The listing builds one solid part. Answer for the finished solid, in the listing's coordinates (mm). Face numbers are marked on the shaded views. A direction names the side the tool comes from. Coordinates: 2 decimals unless noted, no trailing zeros. Order: outer loops, then holes, each group sorted by start corner. A loop starts at its lowest first (then second) coordinate and runs counter-clockwise, first axis right, second up. Notation, with made-up numbers: (19.25, 31.25) -> (49.25, 31.25) arc R10 cw to (49.25, 40.25) -> close; hole circle Ø2 at (1, 1.5). An arc over 180 degrees is marked (long way). Return JSON: item names as keys, results as strings.
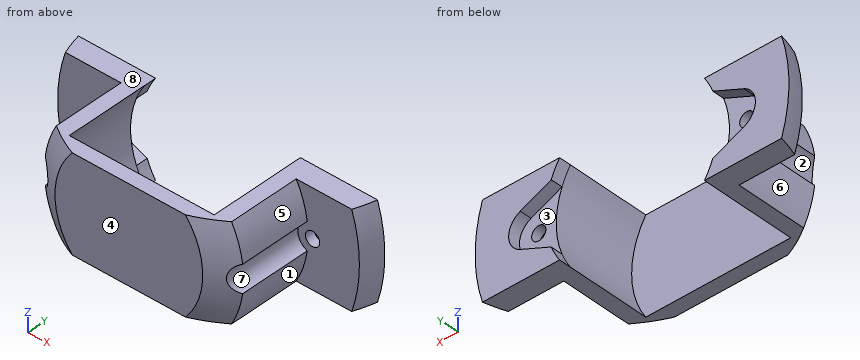
```python
from build123d import *

# Parameters (mm, degrees)
SKETCH2_R               = 33.8
CUT_EXTRUDE1_DEPTH      = 7
SKETCH3_OUTSIDE_W       = 87.592
SKETCH3_OUTSIDE_H       = 87.592
SKETCH3_OUTSIDE_W_2     = 66.134408594
SKETCH3_OUTSIDE_H_2     = 20
CUT_EXTRUDE2_DEPTH      = 54.899165114
CUT_EXTRUDE3_DEPTH      = 2.5
SKETCH6_R               = 18.25
SKETCH6_R_2             = 1.5
CUT_EXTRUDE4_DEPTH      = 17.5
CUT_EXTRUDE5_START      = -19.484712572
CUT_EXTRUDE5_DEPTH      = 14.984712572
CUT_EXTRUDE6_START      = -3
SKETCH8_R               = 33.067204297
CUT_EXTRUDE6_DEPTH      = 37.917915802
CUT_EXTRUDE7_REACH      = 41.188
CUT_EXTRUDE7_END_RADIUS = 33.8
SKETCH9_R               = 3.1


# Read off the part's stored shape, not the designer's step: Cut-Extrude5
with BuildPart() as part:
    # Sketch1 → Revolve1 (revolve)
    with BuildSketch(Plane.XY, mode=Mode.PRIVATE) as revolve1_sk:
        with BuildLine():
            Line((0, -33.8), (0, 0))
            Line((0, 0), (33.8, 0))
            ThreePointArc((33.8, 0), (23.900209204, -23.900209204), (0, -33.8))
        make_face()
    revolve(revolve1_sk.sketch.rotate(Axis((0, -33.8, 0), (0, 1, 0)), 180), axis=Axis((0, -33.8, 0), (0, 1, 0)))

    # Sketch2 → Cut-Extrude1 (cut)
    with BuildSketch(Plane(origin=(0, 0, 0), x_dir=(1, 0, 0), z_dir=(0, 1, 0))):
        Circle(SKETCH2_R)
    extrude(amount=-CUT_EXTRUDE1_DEPTH, mode=Mode.SUBTRACT)

    # Sketch3 outside → Cut-Extrude2 (cut, through all)
    with BuildSketch(Plane(origin=(0, -7, 0), x_dir=(1, 0, 0), z_dir=(0, 1, 0))):
        Rectangle(SKETCH3_OUTSIDE_W, SKETCH3_OUTSIDE_H)
        Rectangle(SKETCH3_OUTSIDE_W_2, SKETCH3_OUTSIDE_H_2, mode=Mode.SUBTRACT)
    extrude(amount=-CUT_EXTRUDE2_DEPTH, mode=Mode.SUBTRACT)

    # Sketch5 → Cut-Extrude3 (cut)
    with BuildSketch(Plane(origin=(0, -7, 0), x_dir=(1, 0, 0), z_dir=(0, 1, 0))):
        with BuildLine():
            Line((-17.025732229, 6.571677263), (-23.544283672, 3.742739979))
            ThreePointArc((-23.544283672, 3.742739979), (-26, 0), (-23.544283672, -3.742739979))
            Line((-23.544283672, -3.742739979), (-17.025732229, -6.571677263))
            ThreePointArc((-17.025732229, -6.571677263), (0, -18.25), (17.025732229, -6.571677263))
            Line((17.025732229, -6.571677263), (23.544283672, -3.742739979))
            ThreePointArc((23.544283672, -3.742739979), (26, 0), (23.544283672, 3.742739979))
            Line((23.544283672, 3.742739979), (17.025732229, 6.571677263))
            ThreePointArc((17.025732229, 6.571677263), (0, 18.25), (-17.025732229, 6.571677263))
        make_face()
    extrude(amount=-CUT_EXTRUDE3_DEPTH, mode=Mode.SUBTRACT)

    # Sketch6 → Cut-Extrude4 (cut)
    with BuildSketch(Plane(origin=(0, -9.5, 0), x_dir=(1, 0, 0), z_dir=(0, 1, 0))):
        Circle(SKETCH6_R)
        with Locations(Location((-21.92, 0, 0), (0, 0, 270))):
            Circle(SKETCH6_R_2)
        with Locations(Location((21.92, 0, 0), (0, 0, 270))):
            Circle(SKETCH6_R_2)
    extrude(amount=-CUT_EXTRUDE4_DEPTH, mode=Mode.SUBTRACT)

    # Cut-Extrude5 outline → Cut-Extrude5 (cut)
    with BuildSketch(Plane(origin=(0, -7, 0), x_dir=(1, 0, 0), z_dir=(0, 1, 0)).offset(CUT_EXTRUDE5_START)):
        with BuildLine():
            ThreePointArc((20.967983577, -1.159165532), (20.206521411, -5.718084686), (18.466185313, -10))
            Line((18.466185313, -10), (33, -10))
            Line((33, -10), (33, 10))
            Line((33, 10), (18.466185313, 10))
            ThreePointArc((18.466185313, 10), (20.206521411, 5.718084686), (20.967983577, 1.159165532))
            ThreePointArc((20.967983577, 1.159165532), (23.42, 0), (20.967983577, -1.159165532))
        make_face()
        with BuildLine():
            ThreePointArc((-18.466185313, -10), (-20.206521411, -5.718084686), (-20.967983577, -1.159165532))
            ThreePointArc((-20.967983577, -1.159165532), (-23.42, 0), (-20.967983577, 1.159165532))
            ThreePointArc((-20.967983577, 1.159165532), (-20.206521411, 5.718084686), (-18.466185313, 10))
            Line((-18.466185313, 10), (-33, 10))
            Line((-33, 10), (-33, -10))
            Line((-33, -10), (-18.466185313, -10))
        make_face()
    extrude(amount=CUT_EXTRUDE5_DEPTH, mode=Mode.SUBTRACT)

    # Sketch8 → Cut-Extrude6 (cut, through all)
    with BuildSketch(Plane(origin=(0, -27, 0), x_dir=(1, 0, 0), z_dir=(0, 1, 0)).offset(CUT_EXTRUDE6_START)):
        Circle(SKETCH8_R)
    extrude(amount=-CUT_EXTRUDE6_DEPTH, mode=Mode.SUBTRACT)

    # Cut-Extrude7: up to this sphere (the profile starts inside it)
    cut_extrude7_end = Location((0, 0, 0)) * Sphere(CUT_EXTRUDE7_END_RADIUS, mode=Mode.PRIVATE)
    # Sketch9 → Cut-Extrude7 (cut, up to the surface)
    with BuildSketch(Plane.XZ.offset(11.5), mode=Mode.PRIVATE) as cut_extrude7_sk1:
        with Locations((-21.92, 0)):
            Circle(SKETCH9_R)
    cut_extrude7_tool1 = extrude(cut_extrude7_sk1.sketch, amount=CUT_EXTRUDE7_REACH, mode=Mode.PRIVATE) & cut_extrude7_end
    add(cut_extrude7_tool1.solids().sort_by_distance((-21.92, -11.5, 0))[0], mode=Mode.SUBTRACT)
    # Sketch9 → Cut-Extrude7 (cut, up to the surface)
    with BuildSketch(Plane.XZ.offset(11.5), mode=Mode.PRIVATE) as cut_extrude7_sk2:
        with Locations((21.92, 0)):
            Circle(SKETCH9_R)
    cut_extrude7_tool2 = extrude(cut_extrude7_sk2.sketch, amount=CUT_EXTRUDE7_REACH, mode=Mode.PRIVATE) & cut_extrude7_end
    add(cut_extrude7_tool2.solids().sort_by_distance((21.92, -11.5, 0))[0], mode=Mode.SUBTRACT)


solid = part.part
```
Item 1: Determine the mould class of the marked faces 6, 7 and 8 for opening direction Z: pulls with the +Z half, pulls with the -Z half, needs draft (parallel to the pull), parting line crosses it, or undercut.
Answer list:
{"face 6": "pulls with the -Z half", "face 7": "undercut", "face 8": "pulls with the +Z half"}
Item 2: The part is cut by section C-C on x = 21.92. Determine the outline of the cut face in (y, z).
Answer list:
{"outline": "(-11.5, -10) -> (-7, -10) -> (-7, -4.45) -> (-9.5, -4.45) -> (-9.5, -1.5) -> (-11.5, -1.5) -> close; (-11.5, 1.5) -> (-9.5, 1.5) -> (-9.5, 4.45) -> (-7, 4.45) -> (-7, 10) -> (-11.5, 10) -> close"}
Item 3: The part is cut by section D-D on z = -4.75. Determine the outline of the cut face in (x, y), plus the area to 3 significant figures.
Answer list:
{"outline": "(-32.72, -7) arc R33.46 ccw to (-31.43, -11.5) -> (-20.46, -11.5) -> (-20.46, -26.48) arc R33.46 ccw to (-14.83, -30) -> (14.83, -30) arc R33.46 ccw to (20.46, -26.48) -> (20.46, -11.5) -> (31.43, -11.5) arc R33.46 ccw to (32.72, -7) -> (21.22, -7) -> (21.22, -9.5) -> (17.62, -9.5) -> (17.62, -27) -> (-17.62, -27) -> (-17.62, -9.5) -> (-21.22, -9.5) -> (-21.22, -7) -> close", "area": "305 mm2"}
Item 4: The part is cut by section B-B on z = 0. Determine the outline of the cut face in (x, y), plus the area to 3 significant figures.
Answer list:
{"outline": "(-33.07, -7) arc R33.8 ccw to (-31.78, -11.5) -> (-23.42, -11.5) -> (-23.42, -9.5) -> (-26, -9.5) -> (-26, -7) -> close; (-20.42, -11.5) -> (-18.82, -11.5) -> (-18.82, -28.08) arc R33.8 ccw to (-15.57, -30) -> (15.57, -30) arc R33.8 ccw to (18.82, -28.08) -> (18.82, -11.5) -> (20.42, -11.5) -> (20.42, -9.5) -> (18.25, -9.5) -> (18.25, -27) -> (-18.25, -27) -> (-18.25, -9.5) -> (-20.42, -9.5) -> close; (23.42, -11.5) -> (31.78, -11.5) arc R33.8 ccw to (33.07, -7) -> (26, -7) -> (26, -9.5) -> (23.42, -9.5) -> close", "area": "202 mm2"}
Item 5: Flat-ended cylindrical pins translate along their axes: pin 1 (10 mm diameter, centred on x = 25, z = 7, fed in from -Y); pin 2 (2.5 mm diameter, centred on x = 21, z = -0.5, fed in from +Y); pin 3 (5 mm diameter, centred on y = -15.5, z = 7, fed in from -X); pin 4 (2 mm diameter, centred on x = 2, y = -24.5, fed in from +Z). Find the tip coordinate at first contact, or state that the pin passes through.
Answer list:
{"pin 1": "y = -26.52", "pin 2": "y = -9.5", "pin 3": "x = -20.51", "pin 4": "through"}
Item 6: The part is cut by section A-A on y = -19.75. Determine the outline of the cut face in (x, z).
Answer list:
{"outline": "(-20.8, -2.89) arc R21 ccw to (-18.47, -10) -> (-15.27, -10) arc R18.25 cw to (-15.27, 10) -> (-18.47, 10) arc R21 ccw to (-20.8, 2.89) arc R3.1 cw to start; (15.27, -10) -> (18.47, -10) arc R21 ccw to (20.8, -2.89) arc R3.1 cw to (20.8, 2.89) arc R21 ccw to (18.47, 10) -> (15.27, 10) arc R18.25 cw to start"}
Item 7: Which of the six approach directions +Z, -Z, +X, -X, +Y, -Y give full straight-line access (tool end or side, diameter ignored) to the marked faces 1, 2, 3, 4 and 5?
Answer list:
{"face 1": "-Z, +X, -Y", "face 2": "-X, -Y", "face 3": "+Y", "face 4": "+Z, -Z, +X, -X, -Y", "face 5": "+Z, +X, -Y"}
Item 8: Find the intervals of material crossed by probe 1 along Z at (x, y) = (-21.92, -10.7); probe 2 along X at (y, z) = (-11, 0); probe 3 along Y at (x, z) = (11, -7), in increasing order.
Answer list:
{"probe 1": "-10 to -1.5, 1.5 to 10", "probe 2": "-31.96 to -23.42, -20.42 to -18.25, 18.25 to 20.42, 23.42 to 31.96", "probe 3": "-30 to -27"}
